Input: dimensioned drawing with shaded views. Units: mm. Origin: part minimum x, y, z. A direction names the side the tool comes from. Round coordinates to 2 decimals unless told otherwise and drop trailing zeros. Order: outer loops, then holes, each group sorted by start corner. A loop starts at its lowest first (then second) coordinate and runs counter-clockwise, first axis right, second up. Notation, with made-up numbers: M -2.75,-5 L 51.25,-5 A21 cw 51.25,13 Z; hole C 75.25,66 d11. An arc over 180 degrees is marked long. One line per question, with ' | ' between items.
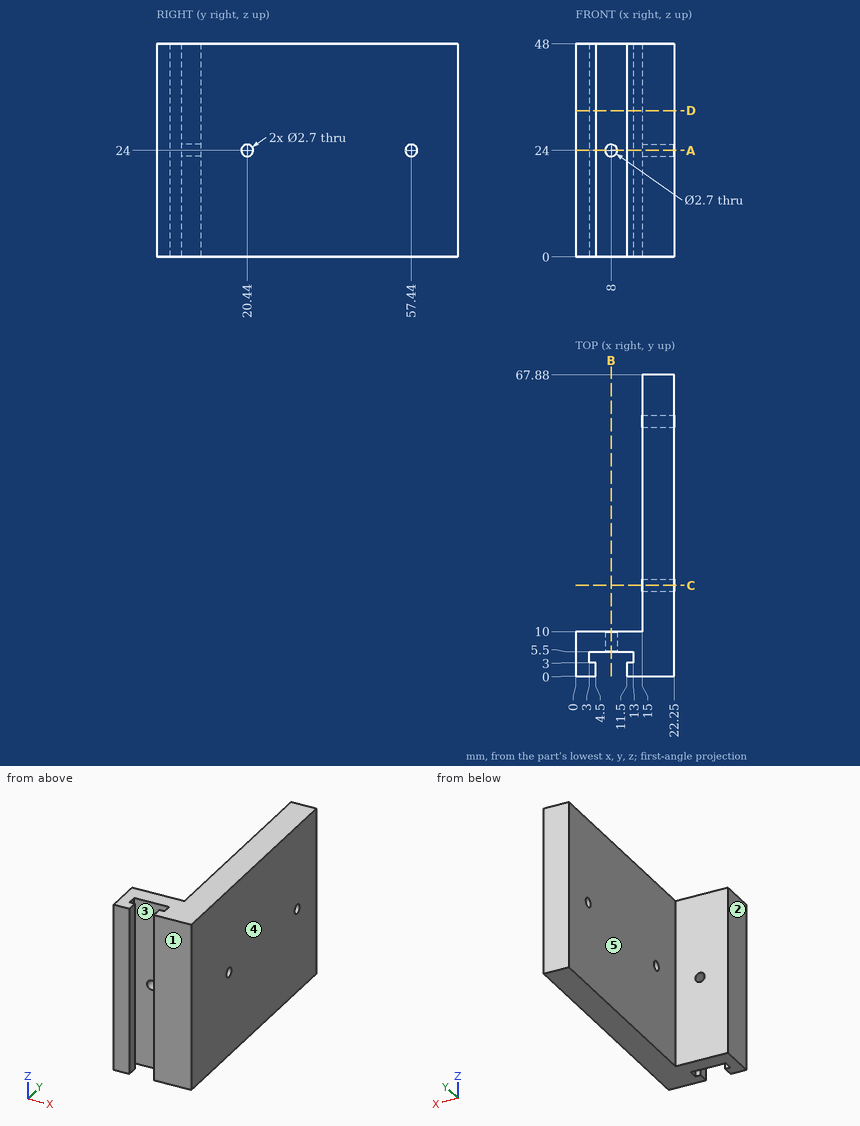
Item 1: Mould query, pull axis X, two halves, no side actions, for the marked faces 1, 2 and 3. Classes: +X half, -X half, draft (parallel to the pull), parting line (faces both ways), or undercut.
Report:
face 1: draft | face 2: -X half | face 3: undercut
Item 2: Line query: line 1 along Y through (x, z) = (20.5, 24); line 2 along Y through (x, z) = (17.25, 23.5); line 3 along Y through (x, z) = (4.25, 24). Output: solid intervals per line, ascending. Write a range as from..to.
Report:
line 1: 0..19.09, 21.79..56.09, 58.79..67.88 | line 2: 0..19.19, 21.69..56.19, 58.69..67.88 | line 3: 0..3, 5.5..10
Item 3: Section query B-B, the plane x = 8. Return loops of the section in (y, z), plus the area to 3 significant figures.
Report:
outline: M 5.5,0 L 10,0 L 10,22.65 L 5.5,22.65 Z; M 5.5,25.35 L 10,25.35 L 10,48 L 5.5,48 Z | area: 204 mm²
Item 4: Section query C-C, the plane y = 20.44. Return loops of the section in (x, z), plus the area to 3 significant figures.
Report:
outline: M 15,0 L 22.25,0 L 22.25,22.65 L 15,22.65 Z; M 15,25.35 L 22.25,25.35 L 22.25,48 L 15,48 Z | area: 328 mm²
Item 5: Access query for the marked faces 4 and 5. Directions: +Z, -Z, +X, -X, +Y, -Y. A direction counts if a zero-diameter tool reaches every point of the face in a straight line with its end or side. Return the directions, or none.
Report:
face 4: +Z, -Z, +X, +Y, -Y | face 5: +Z, -Z, -X, +Y
Item 6: Section query D-D, the plane z = 33. Return loops of the section in (x, y).
Report:
outline: M 0,0 L 4.5,0 L 4.5,3 L 3,3 L 3,5.5 L 13,5.5 L 13,3 L 11.5,3 L 11.5,0 L 22.25,0 L 22.25,67.88 L 15,67.88 L 15,10 L 0,10 Z
Item 7: First-contact query: pin 1 (4.5 mm diameter, centred on y = 20.44, z = 24, fed in from -X); pin 2 (0.8 mm diameter, centred on x = 12, z = 23, fed in from +Y); pin 3 (2.5 mm diameter, centred on x = 8, z = 24, fed in from -Y). Flat tips, straight axial feed; report the tip coordinate or a pass-through.
Report:
pin 1: x = 15 | pin 2: y = 10 | pin 3: through
Item 8: Section query A-A, the plane z = 24. Return loops of the section in (x, y).
Report:
outline: M 0,0 L 4.5,0 L 4.5,3 L 3,3 L 3,5.5 L 6.65,5.5 L 6.65,10 L 0,10 Z; M 9.35,5.5 L 13,5.5 L 13,3 L 11.5,3 L 11.5,0 L 22.25,0 L 22.25,19.09 L 15,19.09 L 15,10 L 9.35,10 Z; M 15,21.79 L 22.25,21.79 L 22.25,56.09 L 15,56.09 Z; M 15,58.79 L 22.25,58.79 L 22.25,67.88 L 15,67.88 Z
